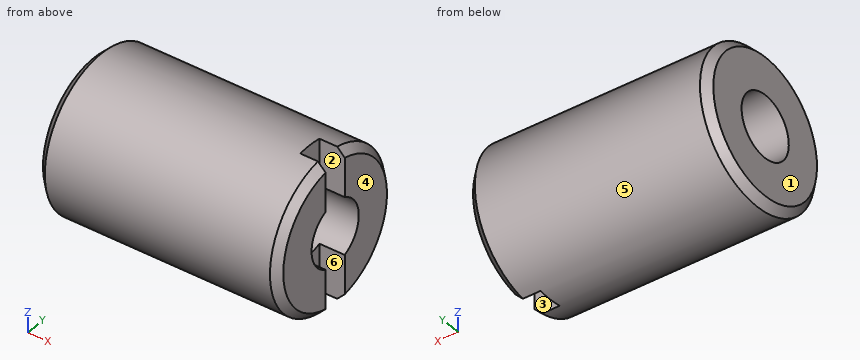
Autodesk Inventor part; units mm, degrees
ref_plane "YZ Plane" through (0, 0, 0) normal (1, 0, 0) x (0, 1, 0)
ref_plane "XZ Plane" through (0, 0, 0) normal (0, 1, 0) x (-1, 0, 0)
ref_plane "XY Plane" through (0, 0, 0) normal (0, 0, 1) x (1, 0, 0)
sketch "スケッチ1" plane through (0, 0, 0) normal (0, 1, 0) x (-1, 0, 0)
  line L0 (0, 0) -> (9.5, 0)
  line L1 (9.5, 0) -> (9.5, -3)
  line L2 (9.5, -3) -> (0, -3)
  line L3 (0, -3) -> (0, 0)
  dimension "d0" = 9.5
  dimension "d1" = 3
revolve "回転1" add sketch "スケッチ1" angle 360 about axis through (0, 0, 0) along (-1, 0, 0)
sketch "スケッチ2" plane through (0, 0, 0) normal (1, 0, 0) x (0, 0, -1)
  point P0 (0, 0)
  point P1 (0, 0)
hole "穴1" at (0, 0, 0) direction (-1, 0, 0) diameter 2.459 end through all
sketch "スケッチ3" plane through (0, 0, 0) normal (1, 0, 0) x (0, 0, -1)
  circle A0 centre (0, 0) radius 3
  line L0 (3, 0) -> (-3, 0)
  line L1 (3, -0.5) -> (-3, -0.5)
  line L2 (3, 0.5) -> (-3, 0.5)
  line L3 (3, 0.5) -> (3, -0.5)
  line L4 (-3, 0.5) -> (-3, -0.5)
  point P0 (-2.958, -0.5)
  point P1 (2.958, -0.5)
  point P2 (2.958, 0.5)
  point P3 (-2.958, 0.5)
  dimension "d10" = 0.5
extrude "押し出し1" cut sketch "スケッチ3" against normal blind 1 contours L0 A0 L2 | A0 L1 L0
chamfer "面取り1" distance 0.3 angle 45 3 edges at (-9.5, 0, 3) (0, 3, 0) (0, -3, 0)
properties part number "ARU-309_5S" material "ステンレス鋼 AISI 304"
Verification items for the finished model (mm, model axes). Face numbers are marked on the shaded views. A direction names the side the tool comes from. Coordinates: 2 decimals unless noted, no trailing zeros. Order: outer loops, then holes, each group sorted by start corner. A loop starts at its lowest first (then second) coordinate and runs counter-clockwise, first axis right, second up. Notation, with made-up numbers: M 80.5,26 L 94.5,26 A23 cw 94.5,34 Z; hole C 37.5,31 d8. An arc over 180 degrees is marked long. Return JSON: item names as keys, results as strings.
1) Cross-section at B-B, the plane y = 0. Record the boundary of the cut face in (x, z).
Answer list:
{"outline": "M -9.5,-2.7 L -9.2,-3 L -1,-3 L -1,-1.23 L -9.5,-1.23 Z; M -9.5,1.23 L -1,1.23 L -1,3 L -9.2,3 L -9.5,2.7 Z"}
2) Access from +Z, -Z, +X, -X, +Y, -Y to the whole of each face (thin tool, end or side, straight path). Record for the marked faces 1 and 2.
Answer list:
{"face 1": "+Z, -Z, -X, +Y, -Y", "face 2": "+Z, -Z, +X"}
3) Thickness scan on L1, parallel to Z at x = -5, y = 0; L2, parallel to Y at x = -9, z = -0.5. Record the ranges inside material, lowest first. Write a range as [from, to].
Answer list:
{"L1": "[-3, -1.23], [1.23, 3]", "L2": "[-2.96, -1.12], [1.12, 2.96]"}
4) Release check for a two-part mould opening along Y. For the marked faces 3, 4, 5 and 6 record: +Y half, -Y half, draft (parallel to the pull), parting line (faces both ways), or undercut.
Answer list:
{"face 3": "undercut", "face 4": "draft", "face 5": "parting line", "face 6": "undercut"}
5) Gauge pin test, flat ends, axial feed: pin 1 (0.5 mm diameter, centred on x = -0.5, z = -2.5, fed in from -Y); pin 2 (0.5 mm diameter, centred on x = -0.5, z = -2.5, fed in from +Y); pin 3 (0.8 mm diameter, centred on y = 0, z = 2.5, fed in from +X). Record the tip position at first contact, or that the pin passes through.
Answer list:
{"pin 1": "y = -1.98", "pin 2": "y = 1.98", "pin 3": "x = -1"}
6) Cross-section at A-A, the plane z = 0. Record the boundary of the cut face in (x, y), and give its area (3 significant figures).
Answer list:
{"outline": "M -9.5,-2.7 L -9.2,-3 L -0.3,-3 L 0,-2.7 L 0,-1.23 L -9.5,-1.23 Z; M -9.5,1.23 L 0,1.23 L 0,2.7 L -0.3,3 L -9.2,3 L -9.5,2.7 Z", "area": "33.5 mm2"}
7) Cross-section at C-C, the plane x = -3.25. Record the boundary of the cut face in (y, z), and give its area (3 significant figures).
Answer list:
{"outline": "C 0,0 d6; hole C 0,0 d2.46", "area": "23.5 mm2"}
